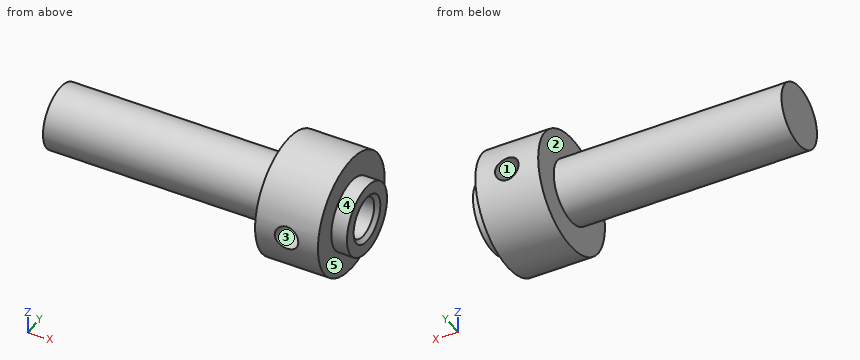
Autodesk Inventor part; units mm, degrees
ref_plane "YZ Plane" through (0, 0, 0) normal (1, 0, 0) x (0, 1, 0)
ref_plane "XZ Plane" through (0, 0, 0) normal (0, 1, 0) x (-1, 0, 0)
ref_plane "XY Plane" through (0, 0, 0) normal (0, 0, 1) x (1, 0, 0)
sketch "Sketch1" plane through (0, 0, 0) normal (0, 0, 1) x (1, 0, 0)
  line L0 (0, 0) -> (0, 4)
  line L1 (0, 4) -> (29, 4)
  line L2 (29, 4) -> (29, 7.5)
  line L3 (29, 7.5) -> (37, 7.5)
  line L4 (37, 7.5) -> (37, 4.5)
  line L5 (37, 4.5) -> (39, 4.5)
  line L6 (39, 4.5) -> (39, 2.5)
  line L7 (39, 2.5) -> (15, 2.5)
  line L8 (15, 2.5) -> (15, 0)
  line L9 (15, 0) -> (0, 0)
  line L10 (0, 0) -> (32.1678, 0)
  dimension "d0" = 8
  dimension "d1" = 39
  dimension "d2" = 15
  dimension "d3" = 8
  dimension "d4" = 2
  dimension "d5" = 9
  dimension "d6" = 5
  dimension "d7" = 15
revolve "Revolution1" add sketch "Sketch1" angle 360 about axis through (0, 0, 0) along (1, 0, 0)
chamfer "Chamfer1" distance 0.5 angle 45 1 edges at (39, -2.5, 0)
sketch "Sketch2" plane through (0, 0, 0) normal (0, 1, 0) x (-1, 0, 0)
  circle A0 centre (-33, 0) radius 1.5
  line L0 (0, -4) -> (-29, -4)
  line L1 (-29, -4) -> (-29, -7.5)
  line L2 (-29, -7.5) -> (-37, -7.5)
  line L3 (-37, -7.5) -> (-37, -4.5)
  line L4 (-37, -4.5) -> (-39, -4.5)
  line L5 (-39, -4.5) -> (-39, -3)
  line L6 (-39, -3) -> (-38.5, -2.5)
  line L7 (-38.5, -2.5) -> (-15, -2.5)
  line L8 (-15, -2.5) -> (-15, 2.5)
  line L9 (-15, 2.5) -> (-38.5, 2.5)
  line L10 (-38.5, 2.5) -> (-39, 3)
  line L11 (-39, 3) -> (-39, 4.5)
  line L12 (-39, 4.5) -> (-37, 4.5)
  line L13 (-37, 4.5) -> (-37, 7.5)
  line L14 (-37, 7.5) -> (-29, 7.5)
  line L15 (-29, 7.5) -> (-29, 4)
  line L16 (-29, 4) -> (0, 4)
  line L17 (0, 4) -> (0, -4)
  line L18 (-37, 7.5) -> (-37, -7.5)
  line L19 (-29, 7.5) -> (-29, -7.5)
  line L20 (-29, 4) -> (-29, -4)
  line L21 (0, 4) -> (0, -4)
  line L22 (-38.5, -2.5) -> (-38.5, 2.5)
  line L23 (0, -4) -> (-29, -4)
  point P0 (0, 0)
  point P1 (-15, 0)
  point P2 (-33, 7.5)
  dimension "d12" = 3
extrude "Extrusion1" cut sketch "Sketch2" along normal through all both and the other way through all contours A0
properties part number "Hjulstopp"
CAD build for the part. Positions are in the model's coordinates, mm. Face numbers are marked on the shaded views. A direction names the side the tool comes from. Round coordinates to 2 decimals unless told otherwise and drop trailing zeros. Order: outer loops, then holes, each group sorted by start corner. A loop starts at its lowest first (then second) coordinate and runs counter-clockwise, first axis right, second up.
Item 1: Probe line 1 along Z through (x, y) = (24.25, 0); line 2 along Z through (x, y) = (29.75, 0); line 3 along X through (y, z) = (5.5, 2). List the from-to ranges inside material, lowest first.
Item 2: Saw through at C-C on x = 33. Write the cut outline in (y, z), then the cut area to 3 significant figures.
Item 3: Tool access for the marked faces 1 and 2: list every direction of +Z, -Z, +X, -X, +Y, -Y with a clear straight run to the whole face (end or side of a thin tool).
Item 4: Saw through at B-B on y = 0. Write the cut outline in (x, z), then the cut area to 3 significant figures.
Item 5: Mould opens along X. For the marked faces 3, 4 and 5 say: pulls with the +X half, pulls with the -X half, needs draft (parallel to the pull), parting line crosses it, or undercut.
Item 6: Saw through at A-A on z = 0. Write the cut outline in (x, y), then the cut area to 3 significant figures.
Item 7: Pin check, flat tips, straight feed: pin 1 (1.5 mm diameter, centred on y = 1, z = 0, fed in from +X); pin 2 (4 mm diameter, centred on y = -5, z = 4.5, fed in from -X); pin 3 (3 mm diameter, centred on x = 25, z = 4.5, fed in from +Y). Stop position of each tip, or through.
Item 8: Saw through at D-D on x = 13.5. Write the cut outline in (y, z), then the cut area to 3 significant figures.
Reported:
1. line 1: z = -4 to -2.5, 2.5 to 4
1. line 2: z = -7.5 to -2.5, 2.5 to 7.5
1. line 3: x = 29 to 37
2. outline: (-7.35, -1.5) arc R7.5 ccw to (7.35, -1.5) - (2, -1.5) arc R2.5 cw to (-2, -1.5) - close; (-7.35, 1.5) - (-2, 1.5) arc R2.5 cw to (2, 1.5) - (7.35, 1.5) arc R7.5 ccw to start
2. area: 126 mm2
3. face 1: +Y, -Y
3. face 2: -X
4. outline: (0, -4) - (29, -4) - (29, -7.5) - (37, -7.5) - (37, -4.5) - (39, -4.5) - (39, -3) - (38.5, -2.5) - (15, -2.5) - (15, 2.5) - (38.5, 2.5) - (39, 3) - (39, 4.5) - (37, 4.5) - (37, 7.5) - (29, 7.5) - (29, 4) - (0, 4) - close
4. area: 250 mm2
5. face 3: undercut
5. face 4: needs draft
5. face 5: pulls with the +X half
6. outline: (0, -4) - (29, -4) - (29, -7.5) - (31.5, -7.5) - (31.5, -2.5) - (15, -2.5) - (15, 2.5) - (31.5, 2.5) - (31.5, 7.5) - (29, 7.5) - (29, 4) - (0, 4) - close; (34.5, -7.5) - (37, -7.5) - (37, -4.5) - (39, -4.5) - (39, -3) - (38.5, -2.5) - (34.5, -2.5) - close; (34.5, 2.5) - (38.5, 2.5) - (39, 3) - (39, 4.5) - (37, 4.5) - (37, 7.5) - (34.5, 7.5) - close
6. area: 220 mm2
7. pin 1: stops at x = 15
7. pin 2: stops at x = 29
7. pin 3: stops at y = 2.65
8. outline: circle Ø8 at (0, 0)
8. area: 50.3 mm2
